```python
from build123d import *

# Parameters (mm, degrees)
SKETCH2_R           = 75
BOSS_EXTRUDE2_DEPTH = 5
SKETCH3_R           = 20
CUT_EXTRUDE2_DEPTH  = 107.183802908
FILLET2_R           = 10
FILLET3_R           = 5


with BuildPart() as part:
    # Sketch2 → Boss-Extrude2 (new body)
    with BuildSketch(Plane(origin=(0, 0, 0), x_dir=(1, 0, 0), z_dir=(0, 1, 0))):
        with Locations(Location((0, 0, 0), (0, 0, 270))):
            Circle(SKETCH2_R)
    extrude(amount=BOSS_EXTRUDE2_DEPTH)

    # Sketch3 → Cut-Extrude2 (cut, through all)
    with BuildSketch(Plane(origin=(0, 5, 0), x_dir=(1, 0, 0), z_dir=(0, 1, 0))):
        with Locations((0, 56)):
            Circle(SKETCH3_R)
        with Locations((48.497422612, -28)):
            Circle(SKETCH3_R)
        with Locations((-48.497422612, -28)):
            Circle(SKETCH3_R)
    extrude(amount=-CUT_EXTRUDE2_DEPTH, mode=Mode.SUBTRACT)

    # Fillet2
    fillet2_edges = [part.edges().sort_by_distance(p)[0] for p in [
        (7.218787271, 2.5, -74.651785714),
        (61.040949231, 2.5, 43.577546019),
        (-68.259736502, 2.5, 31.074239696),
    ]]
    fillet(fillet2_edges, radius=FILLET2_R)

    # Fillet3
    fillet3_edges = [part.edges().sort_by_distance(p)[0] for p in [
        (-7.218787271, 2.5, -74.651785714),
        (68.259736502, 2.5, 31.074239696),
        (-61.040949231, 2.5, 43.577546019),
    ]]
    fillet(fillet3_edges, radius=FILLET3_R)


solid = part.part
```
CAD build for the part. Positions are in the model's coordinates, mm. Coordinates: 2 decimals unless noted, no trailing zeros. Write each loop counter-clockwise with the first axis right and the second up, starting at its lowest first coordinate (ties: lowest second). Pieces come first, ordered by that corner, then holes.
(1) Flat gauge pin, fed straight in: pin 1 (2 mm diameter, centred on y = 1, z = -54, fed in from -X). Where does the tip first touch, or does it go through?
(2) Cut at B-B, the plane x = 0. List the corners of the cut face in (y, z), and give its area (3 significant figures).
(3) Drill centre lines: probe 1 along Z at (x, y) = (0, 3.3); probe 2 along X at (y, z) = (1.9, -59); probe 3 along X at (y, z) = (1.75, 28). Where is each one in solid material? Low to high.
(4) Cut at A-A, the plane z = -49.5. List the corners of the cut face in (x, y).
(5) Two-plate mould, pull along X, no slides. Class faces 1 (the face through (-6.163, 2.465, 74.746)), 2 (the face through (67.81, 2.46, -32.04)), 3 (the face through (-61.65, 2.46, -42.71)), 4 (the face through (-4.104, 2.535, -36.426)): +X half, -X half, draft (parallel to the pull), parting line (faces both ways), or undercut.
(6) Cut at C-C, the plane z = -21. List the corners of the cut face in (x, y).
Geometry says:
1. pin 1: stops at x = -53.07
2. outline: (0, -36) - (5, -36) - (5, 75) - (0, 75) - close
2. area: 555 mm2
3. probe 1: z = -36 to 75
3. probe 2: x = -46.3 to -19.77, 20.04 to 46.3
3. probe 3: x = -28.5 to 28.5
4. outline: (-56.34, 0) - (-18.91, 0) - (-18.91, 5) - (-56.34, 5) - close; (18.91, 0) - (56.34, 0) - (56.34, 5) - (18.91, 5) - close
5. face 1: parting line
5. face 2: +X half
5. face 3: -X half
5. face 4: undercut
6. outline: (-72, 0) - (72, 0) - (72, 5) - (-72, 5) - close
